from build123d import *

# Parameters (mm, degrees)
F0_R     = 14.2875
F1_DEPTH = 19.304
F2_R     = 18.415
F3_DEPTH = 3.81
F4_R     = 18.415
F5_DEPTH = 3.81


with BuildPart() as f1:
    # F0 (on Top) → F1 (new body)
    with BuildSketch(Plane.XY):
        Circle(F0_R)
        Polygon((-3.678436, 6.427525), (3.727182, 6.399382), (7.405618, -0.028143), (3.678436, -6.427525), (-3.727182, -6.399382), (-7.405618, 0.028143), align=None, mode=Mode.SUBTRACT)
    extrude(amount=F1_DEPTH)

    # F2 (on face) → F3 (join)
    with BuildSketch(Plane.XY.offset(19.304)):
        with Locations((0, -0.028143)):
            Circle(F2_R)
        Polygon((-3.678436, 6.427525), (3.727182, 6.399382), (7.405618, -0.028143), (3.678436, -6.427525), (-3.727182, -6.399382), (-7.405618, 0.028143), align=None, mode=Mode.SUBTRACT)
    extrude(amount=F3_DEPTH)

    # F4 (on face) → F5 (join)
    with BuildSketch(Plane(origin=(0, 0, 0), x_dir=(1, 0, 0), z_dir=(0, 0, -1))):
        Circle(F4_R)
        Polygon((3.678436, 6.427525), (7.405618, 0.028143), (3.727182, -6.399382), (-3.678436, -6.427525), (-7.405618, -0.028143), (-3.727182, 6.399382), align=None, mode=Mode.SUBTRACT)
    extrude(amount=F5_DEPTH)


solid = f1.part
Model file for the job. Use its own axes, mm. A direction names the side the tool comes from. Give positions to 0.01 mm unless a question says otherwise; leave off trailing zeros. Order: outer loops, then holes, each group sorted by start corner. A loop starts at its lowest first (then second) coordinate and runs counter-clockwise, first axis right, second up. Notation, with made-up numbers: M -19,9 L 29,9 A33 cw 29,43 Z; hole C -26,82.25 d1. An arc over 180 degrees is marked long. Put each result on its own line as item: value. Start each with the question number.
(1) Tool access for faces 1 (the face through (-14, -4, 19.304)), 2 (the face through (0, -8, 23.114)), 3 (the face through (-5.5, 3.3, 9.8)): list every direction of +Z, -Z, +X, -X, +Y, -Y with a clear straight run to the whole face (end or side of a thin tool).
(2) Pin check, flat tips, straight feed: pin 1 Ø5 at (x, z) = (14.5, 1) entering from -Y; pin 2 Ø6 at (y, z) = (1.5, 14) entering from -X; pin 3 Ø4 at (x, z) = (-4, 8.5) entering from -Y. Stop position of each tip, or through.
(3) Drill centre lines: L1, parallel to Z at x = 13, y = -7.5; L2, parallel to X at y = 3.5, z = 8.25; L3, parallel to Y at x = -1, z = 14. Where is each one in solid material? Low to high. Write a range as [from, to].
(4) Band-saw the part on B-B on y = -3.5. Give the cut face in (x, z).
(5) Band-saw the part on D-D on z = -1.25. Give the cut face in (x, y) (3 decimals), then the cut area to 3 significant figures.
(6) Band-saw the part on C-C on x = -6. Give the cut face in (y, z).
(7) Band-saw the part on A-A on z = 15. Give the cut face in (x, y) (1 decimal), then the cut area to 3 significant figures.
(8) Pull direction Y, two halves, no side cores. Call faces 4 (the face through (-14.274, 0.628, 9.517)), 5 (the face through (5, 14, 0)), 6 (the face through (5.5, -3.3, 9.8)): released by +Y, released by -Y, zero draft, split by the parting line, or undercut.
Results below:
1. face 1: none
1. face 2: +Z, +X, -X, +Y, -Y
1. face 3: +Z, -Z
2. pin 1: stops at y = -13.79
2. pin 2: stops at x = -14.29
2. pin 3: stops at y = -14.15
3. L1: z = [-3.81, 0], [19.3, 23.11]
3. L2: x = [-13.85, -5.38], [5.39, 13.85]
3. L3: y = [-14.25, -6.41], [6.42, 14.25]
4. outline: M -18.08,-3.81 L -5.39,-3.81 L -5.39,23.11 L -18.08,23.11 L -18.08,19.3 L -13.85,19.3 L -13.85,0 L -18.08,0 Z; M 5.38,-3.81 L 18.08,-3.81 L 18.08,0 L 13.85,0 L 13.85,19.3 L 18.08,19.3 L 18.08,23.11 L 5.38,23.11 Z
5. outline: C 0,0 d36.83; hole M -7.406,0.028 L -3.727,-6.399 L 3.678,-6.428 L 7.406,-0.028 L 3.727,6.399 L -3.678,6.428 Z
5. area: 923 mm2
6. outline: M -17.44,19.3 L -12.97,19.3 L -12.97,0 L -17.41,0 L -17.41,-3.81 L -2.43,-3.81 L -2.43,23.11 L -17.44,23.11 Z; M 2.44,-3.81 L 17.41,-3.81 L 17.41,0 L 12.97,0 L 12.97,19.3 L 17.38,19.3 L 17.38,23.11 L 2.44,23.11 Z
7. outline: C 0,0 d28.6; hole M -7.4,0 L -3.7,-6.4 L 3.7,-6.4 L 7.4,0 L 3.7,6.4 L -3.7,6.4 Z
7. area: 499 mm2
8. face 4: split by the parting line
8. face 5: zero draft
8. face 6: undercut
